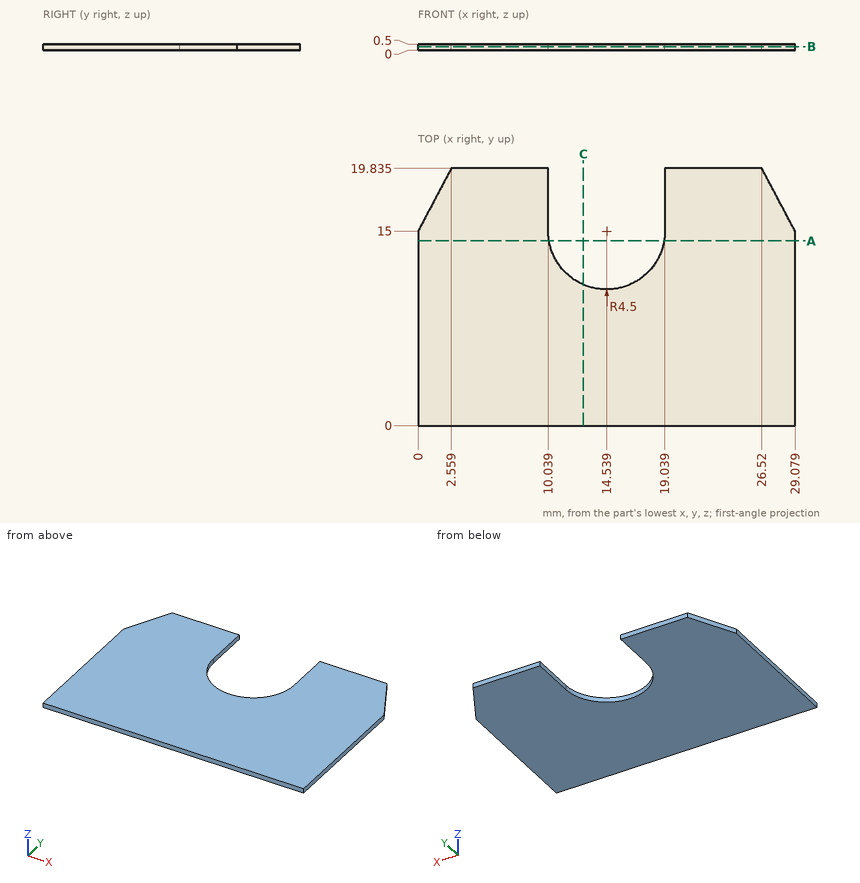
Answer from the drawing. Dimensions are ordinates in mm from the lowest x, y and z of the part. Round coordinates to 2 decimals unless told otherwise and drop trailing zeros. Write each loop counter-clockwise with the first axis right and the second up, starting at its lowest first coordinate (ties: lowest second). Pieces come first, ordered by that corner, then holes.
1. The part is cut by section C-C, the plane x = 12.75. Determine the outline of the cut face in (y, z).
2. The part is cut by section A-A, the plane y = 14.25. Determine the outline of the cut face in (x, z), then the cut area to 3 significant figures.
3. The part is cut by section B-B, the plane z = 0.3. Determine the outline of the cut face in (x, y) (1 decimal).
4. Straight lines are drawn through the part: L1, parallel to X at y = 16.5, z = 0.35 (1 decimal); L2, parallel to X at y = 17.5, z = 0.2 (1 decimal); L3, parallel to Y at x = 11.5, z = 0.25. For each, find the intervals that lie inside material, in ascending order.
Values:
1. outline: (0, 0) - (10.87, 0) - (10.87, 0.5) - (0, 0.5) - close
2. outline: (0, 0) - (10.1, 0) - (10.1, 0.5) - (0, 0.5) - close; (18.98, 0) - (29.08, 0) - (29.08, 0.5) - (18.98, 0.5) - close
2. area: 10.1 mm2
3. outline: (0, 0) - (29.1, 0) - (29.1, 15) - (26.5, 19.8) - (19, 19.8) - (19, 15) arc R4.5 cw to (10, 15) - (10, 19.8) - (2.6, 19.8) - (0, 15) - close
4. L1: x = 0.8 to 10, 19 to 28.3
4. L2: x = 1.3 to 10, 19 to 27.8
4. L3: y = 0 to 11.68
